from build123d import *

# Parameters (mm, degrees)
SKETCH1_W                                         = 17.5
SKETCH1_H                                         = 35
BASE_FLANGE1_DEPTH                                = 2
SKETCH11_R                                        = 4
CUT_EXTRUDE3_DEPTH                                = 2
SKETCHED_START                                    = -23.286713287
SKETCHED_BEND3_DEPTH                              = 17.5
SKETCHED_BEND3_2_DEPTH                            = 4.7499999
SKETCHED_START_2                                  = -10.536713187
SKETCHED_BEND3_3_DEPTH                            = 4.7499999
SKETCHED_START_3                                  = -18.536713387
SKETCHED_BEND3_4_DEPTH                            = 8.0000002
SKETCHED_START_4                                  = -10.59323683
SKETCHED_BEND3_5_OUTLINE_R                        = 4
SKETCHED_BEND3_5_DEPTH                            = 2
CSK_FOR_4_FLAT_HEAD_MACHINE_SCREW_100_D           = 3.2639
CSK_FOR_4_FLAT_HEAD_MACHINE_SCREW_100_DEPTH       = 2
CSK_FOR_4_FLAT_HEAD_MACHINE_SCREW_100_CSINK_D     = 5.715
CSK_FOR_4_FLAT_HEAD_MACHINE_SCREW_100_CSINK_ANGLE = 100
CSK_FOR_4_FLAT_HEAD_MACHINE_SCREW_100_TIP         = 0.980574487


with BuildPart() as part:
    # Base-Flange1: sheet metal written as solids
    # Sketch1 → Base-Flange1 (new body)
    with BuildSketch(Plane(origin=(0, 0, 0), x_dir=(1, 0, 0), z_dir=(0, 1, 0))):
        with Locations((-14.536713287, 3.82983683)):
            Rectangle(SKETCH1_W, SKETCH1_H)
    extrude(amount=-BASE_FLANGE1_DEPTH)

    # Sketch11 → Cut-Extrude3 (cut)
    with BuildSketch(Plane(origin=(0, 0, 0), x_dir=(1, 0, 0), z_dir=(0, 1, 0))):
        with Locations(Location((-14.536713287, -6.17016317, 0), (0, 0, 270))):
            Circle(SKETCH11_R)
    extrude(amount=-CUT_EXTRUDE3_DEPTH, mode=Mode.SUBTRACT)

    # Sketched Bend3: read off the stored shape, not the designer's step
    # Sketched Bend3 outline → Sketched Bend3 (cut)
    with BuildSketch(Plane.YZ.offset(SKETCHED_START)):
        with BuildLine():
            ThreePointArc((-2, -11.32983683), (-1.443395312, -9.675569621), (0, -8.694234432))
            Line((0, -8.694234432), (0, 13.67016317))
            Line((0, 13.67016317), (-2, 13.67016317))
            Line((-2, 13.67016317), (-2, -11.32983683))
        make_face()
    extrude(amount=SKETCHED_BEND3_DEPTH, mode=Mode.SUBTRACT)

    # Sketched Bend3 2 outline → Sketched Bend3 2 (add)
    with BuildSketch(Plane.YZ.offset(SKETCHED_START)):
        with BuildLine():
            ThreePointArc((0, -11.32983683), (0.215745145, -10.808981975), (0.7366, -10.59323683))
            Line((0.7366, -10.59323683), (23.197250658, -10.59323683))
            Line((23.197250658, -10.59323683), (23.197250658, -8.59323683))
            Line((23.197250658, -8.59323683), (0.7366, -8.59323683))
            ThreePointArc((0.7366, -8.59323683), (0.364854094, -8.6186038), (0, -8.694234432))
            Line((0, -8.694234432), (0, -11.32983683))
        make_face()
    extrude(amount=SKETCHED_BEND3_2_DEPTH)

    # Sketched Bend3 3 outline → Sketched Bend3 3 (add)
    with BuildSketch(Plane.YZ.offset(SKETCHED_START_2)):
        with BuildLine():
            ThreePointArc((0, -11.32983683), (0.215745145, -10.808981975), (0.7366, -10.59323683))
            Line((0.7366, -10.59323683), (23.197250658, -10.59323683))
            Line((23.197250658, -10.59323683), (23.197250658, -8.59323683))
            Line((23.197250658, -8.59323683), (0.7366, -8.59323683))
            ThreePointArc((0.7366, -8.59323683), (0.364854094, -8.6186038), (0, -8.694234432))
            Line((0, -8.694234432), (0, -11.32983683))
        make_face()
    extrude(amount=SKETCHED_BEND3_3_DEPTH)

    # Sketched Bend3 4 outline → Sketched Bend3 4 (add)
    with BuildSketch(Plane.YZ.offset(SKETCHED_START_3)):
        with BuildLine():
            ThreePointArc((0, -11.32983683), (0.215745145, -10.808981975), (0.7366, -10.59323683))
            Line((0.7366, -10.59323683), (23.197250658, -10.59323683))
            Line((23.197250658, -10.59323683), (23.197250658, -8.59323683))
            Line((23.197250658, -8.59323683), (0.7366, -8.59323683))
            ThreePointArc((0.7366, -8.59323683), (0.364854094, -8.6186038), (0, -8.694234432))
            Line((0, -8.694234432), (0, -11.32983683))
        make_face()
    extrude(amount=SKETCHED_BEND3_4_DEPTH)

    # Sketched Bend3 5 outline → Sketched Bend3 5 (cut)
    with BuildSketch(Plane.XY.offset(SKETCHED_START_4)):
        with Locations((-14.536713287, 15.697250658)):
            Circle(SKETCHED_BEND3_5_OUTLINE_R)
    extrude(amount=SKETCHED_BEND3_5_DEPTH, mode=Mode.SUBTRACT)

    # CSK for #4 Flat Head Machine Screw (100)2
    with Locations(Plane.XZ.offset(2)):
        with Locations((-9.786713287, -16.32983683), (-19.286713287, -16.32983683)):
            CounterSinkHole(CSK_FOR_4_FLAT_HEAD_MACHINE_SCREW_100_D / 2, CSK_FOR_4_FLAT_HEAD_MACHINE_SCREW_100_CSINK_D / 2, depth=CSK_FOR_4_FLAT_HEAD_MACHINE_SCREW_100_DEPTH, counter_sink_angle=CSK_FOR_4_FLAT_HEAD_MACHINE_SCREW_100_CSINK_ANGLE)
            with Locations((0, 0, -(CSK_FOR_4_FLAT_HEAD_MACHINE_SCREW_100_DEPTH + CSK_FOR_4_FLAT_HEAD_MACHINE_SCREW_100_TIP / 2))):  # 118° drill point
                Cone(0, CSK_FOR_4_FLAT_HEAD_MACHINE_SCREW_100_D / 2, CSK_FOR_4_FLAT_HEAD_MACHINE_SCREW_100_TIP, mode=Mode.SUBTRACT)


solid = part.part
The model under review builds one solid part; all positions refer to its coordinate system, in mm. A direction names the side the tool comes from. Coordinates: 2 decimals unless noted, no trailing zeros. Loops run counter-clockwise (first coordinate to the right, second up) from the corner with the lowest first, then second, coordinate; pieces in that order, holes last. Notation, with made-up numbers: M 6,36 L 46,36 A36 cw 46,71 Z; hole C 47,-39 d7. An arc over 180 degrees is marked long. Put each result on its own line as item: value. Start each with the question number.
Q1. Add section C-C (z = -11). Write out the cut boundary in (x, y), and give its area (3 significant figures).
Q2. Add section D-D (y = 12.75). Write out the cut boundary in (x, z).
Q3. For faces 4 (the flat face through (-17, 12, -10.593)), 5 (the cylindrical face through (-10.72, 16.9, -9.61)), list the 3-axis set-ups (+Z, -Z, +X, -X, +Y, -Y) from which the entire face can be reached by the end or side of a thin tool; tool diameter is ignored.
Q4. Add section B-B (y = 1.75). Write out the cut boundary in (x, z).
Q5. Wall thickness on line 1 (Z direction, x = -22.5, y = 14.5); line 2 (Y direction, x = -14.75, z = -12.25); line 3 (Y direction, x = -22.5, z = -9.5): over which ranges is each line inside the solid? List them lowest first.
Q6. Add section A-A (y = 18.25). Write out the cut boundary in (x, z).
Q7. Clearance check with flat-ended pins moving along their axes: pin 1 (5 mm diameter, centred on x = -14.5, z = -18, fed in from +Y); pin 2 (4 mm diameter, centred on x = -19.29, z = -16.33, fed in from -Y); pin 3 (6 mm diameter, centred on x = -15.5, y = 17, fed in from -Z); pin 4 (7 mm diameter, centred on x = -14.54, y = 15.7, fed in from +Z). State where each tip first meets the part, or that it passes through.
Q8. The part is to be moulded in two halves that separate along X. For faces 1 (the cylindrical face through (-9.433, -0.479, -17.923)), 2 (the flat face through (-5.787, 7, -10)), 3 (the flat face through (-15, -1, -21.33)), say which applies: +X half, -X half, draft (parallel to the pull), parting line (faces both ways), or undercut.
Answers:
1. outline: M -23.29,-1.98 L -5.79,-1.98 L -5.79,0.08 L -23.29,0.08 Z
1. area: 36.0 mm^2
2. outline: M -23.29,-10.59 L -17.24,-10.59 L -17.24,-8.59 L -23.29,-8.59 Z; M -11.83,-10.59 L -5.79,-10.59 L -5.79,-8.59 L -11.83,-8.59 Z
3. face 4: -Z, +X, -X, +Y
3. face 5: +Z, -Z
4. outline: M -23.29,-10.59 L -5.79,-10.59 L -5.79,-8.59 L -23.29,-8.59 Z
5. line 1: z = -10.59 to -8.59
5. line 2: y = -2 to 0
5. line 3: y = -1.3 to 23.2
6. outline: M -23.29,-10.59 L -17.62,-10.59 L -17.62,-8.59 L -23.29,-8.59 Z; M -11.46,-10.59 L -5.79,-10.59 L -5.79,-8.59 L -11.46,-8.59 Z
7. pin 1: stops at y = 0
7. pin 2: stops at y = -1.28
7. pin 3: stops at z = -10.59
7. pin 4: passes through
8. face 1: undercut
8. face 2: +X half
8. face 3: draft
